Verification items for the finished model (mm, model axes). A direction names the side the tool comes from. Give positions to 0.01 mm unless a question says otherwise; leave off trailing zeros. Write each loop counter-clockwise with the first axis right and the second up, starting at its lowest first coordinate (ties: lowest second). Pieces come first, ordered by that corner, then holes. Notation, with made-up numbers: (13, 69) -> (40, 69) arc R16 cw to (40, 74) -> close; hole circle Ø3 at (54.5, 34.5). An arc over 180 degrees is marked (long way). Write item = value, one per line.
from build123d import *

# Parameters (mm, degrees)
F0_W     = 121.92
F0_H     = 24.13
F0_W_2   = 96.52
F0_H_2   = 17.272
F1_DEPTH = 5.08
F2_W     = 135.89
F2_H     = 38.1
F2_W_2   = 121.92
F2_H_2   = 24.13
F3_DEPTH = 21.59


with BuildPart() as f1:
    # F0 (on Front) → F1 (new body)
    with BuildSketch(Plane.XZ):
        Rectangle(F0_W, F0_H)
        Rectangle(F0_W_2, F0_H_2, mode=Mode.SUBTRACT)
    extrude(amount=F1_DEPTH)

    # F2 (on Front) → F3 (join)
    with BuildSketch(Plane.XZ):
        Rectangle(F2_W, F2_H)
        Rectangle(F2_W_2, F2_H_2, mode=Mode.SUBTRACT)
    extrude(amount=F3_DEPTH)


solid = f1.part
Item 1: Sectioned sample at D-D on x = 53.5. Record the cut outline in (y, z) (3 decimals), then the cut area to 3 significant figures.
Response values:
outline = (-21.59, -19.05) -> (0, -19.05) -> (0, 19.05) -> (-21.59, 19.05) -> (-21.59, 12.065) -> (-5.08, 12.065) -> (-5.08, -12.065) -> (-21.59, -12.065) -> close
area = 424 mm^2
Item 2: Sectioned sample at B-B on z = -3.5. Record the cut outline in (x, y) (3 decimals), then the cut area to 3 significant figures.
Response values:
outline = (-67.945, -21.59) -> (-60.96, -21.59) -> (-60.96, -5.08) -> (-48.26, -5.08) -> (-48.26, 0) -> (-67.945, 0) -> close; (48.26, -5.08) -> (60.96, -5.08) -> (60.96, -21.59) -> (67.945, -21.59) -> (67.945, 0) -> (48.26, 0) -> close
area = 431 mm^2
Item 3: Material ranges on line 1 (Z direction, x = -20, y = -9.5) (3 decimals); line 2 (X direction, y = -15.25, z = 6.5) (3 decimals); line 3 (Z direction, x = 13, y = -1.5), recorded low to high.
Response values:
line_1 = -19.05 to -12.065, 12.065 to 19.05
line_2 = -67.945 to -60.96, 60.96 to 67.945
line_3 = -19.05 to -8.64, 8.64 to 19.05
Item 4: Go/stop test with flat-tipped pins: P1, Ø3, axis at x = -16, z = -9.5, coming from the -Y side; P2, Ø4, axis at x = 3.5, z = 11.5, coming from the +Y side. Record where each tip stops, or that it passes through.
Response values:
P1 = -5.08
P2 = 0
Item 5: Set-up check for faces 1 (the flat face through (-48.26, -3, 0)), 2 (the flat face through (-67.945, -11, 0)), 3 (the flat face through (-1, -13, -12.065)): record each of +Z, -Z, +X, -X, +Y, -Y from which the full face is reachable in a straight line by a thin tool's end or side.
Response values:
face_1 = +Y, -Y
face_2 = +Z, -Z, -X, +Y, -Y
face_3 = -Y
Item 6: Mould release check, pull along X, two halves, no side actions. Record for faces 4 (the flat face through (67.945, -11, 0)), 5 (the flat face through (-1, -21.59, 13)), 6 (the flat face through (-60.96, -13, 0)), 7 (the flat face through (-1, -3, -8.636)): +X half, -X half, draft (parallel to the pull), parting line (faces both ways), or undercut.
Response values:
face_4 = +X half
face_5 = draft
face_6 = undercut
face_7 = undercut
Item 7: Sectioned sample at A-A on x = 26.5. Record the cut outline in (y, z) (3 decimals), then the cut area to 3 significant figures.
Response values:
outline = (-21.59, -19.05) -> (0, -19.05) -> (0, -8.636) -> (-5.08, -8.636) -> (-5.08, -12.065) -> (-21.59, -12.065) -> close; (-21.59, 12.065) -> (-5.08, 12.065) -> (-5.08, 8.636) -> (0, 8.636) -> (0, 19.05) -> (-21.59, 19.05) -> close
area = 336 mm^2
Item 8: Sectioned sample at C-C on y = -3.75. Record the cut outline in (x, z) (3 decimals), then the cut area to 3 significant figures.
Response values:
outline = (-67.945, -19.05) -> (67.945, -19.05) -> (67.945, 19.05) -> (-67.945, 19.05) -> close; hole (-48.26, -8.636) -> (48.26, -8.636) -> (48.26, 8.636) -> (-48.26, 8.636) -> close
area = 3,510 mm^2
